Could you check a few things on this drawing? It's one solid part, dimensions in mm from its lowest x, y, z. A direction names the side the tool comes from. Round coordinates to 2 decimals unless told otherwise and drop trailing zeros. Write each loop counter-clockwise with the first axis right and the second up, starting at its lowest first coordinate (ties: lowest second). Pieces come first, ordered by that corner, then holes. Notation, with made-up numbers: (-2.5, 21) -> (11.5, 21) arc R7 cw to (11.5, 26) -> close; hole circle Ø8 at (-22.5, -23.75). An arc over 180 degrees is marked (long way). Put each result on its own line as item: value. Start each with the question number.
1) If I drill on line 1 along Y through (x, z) = (31, 18); line 2 along X through (y, z) = (3.5, 12.5), over which ranges is the centre line in solid material (lowest first)? Write a range as [from, to].
2) I want a section at A-A, the plane y = 8.5. List the corners of the cut face in (x, z) for me, then the cut area to 3 significant figures.
3) I want a section at B-B, the plane z = 12.5. List the corners of the cut face in (x, y) for me.
4) Which directions (+Z, -Z, +X, -X, +Y, -Y) give clear straight access to the entire face, cutting with the end or side of a thin tool? Please do the marked faces 4 and 5.
5) I want a section at D-D, the plane y = 25. List the corners of the cut face in (x, z) for me, then the cut area to 3 significant figures.
6) We'd pull the mould along X, two halves only. Please class the marked faces 1, 2 and 3: released by +X, released by -X, zero draft, split by the parting line, or undercut.
7) Will this pin go through, and if not, where does the flat tip stop? P1, Ø1, axis at x = 36, z = 6, coming from the -Y side.
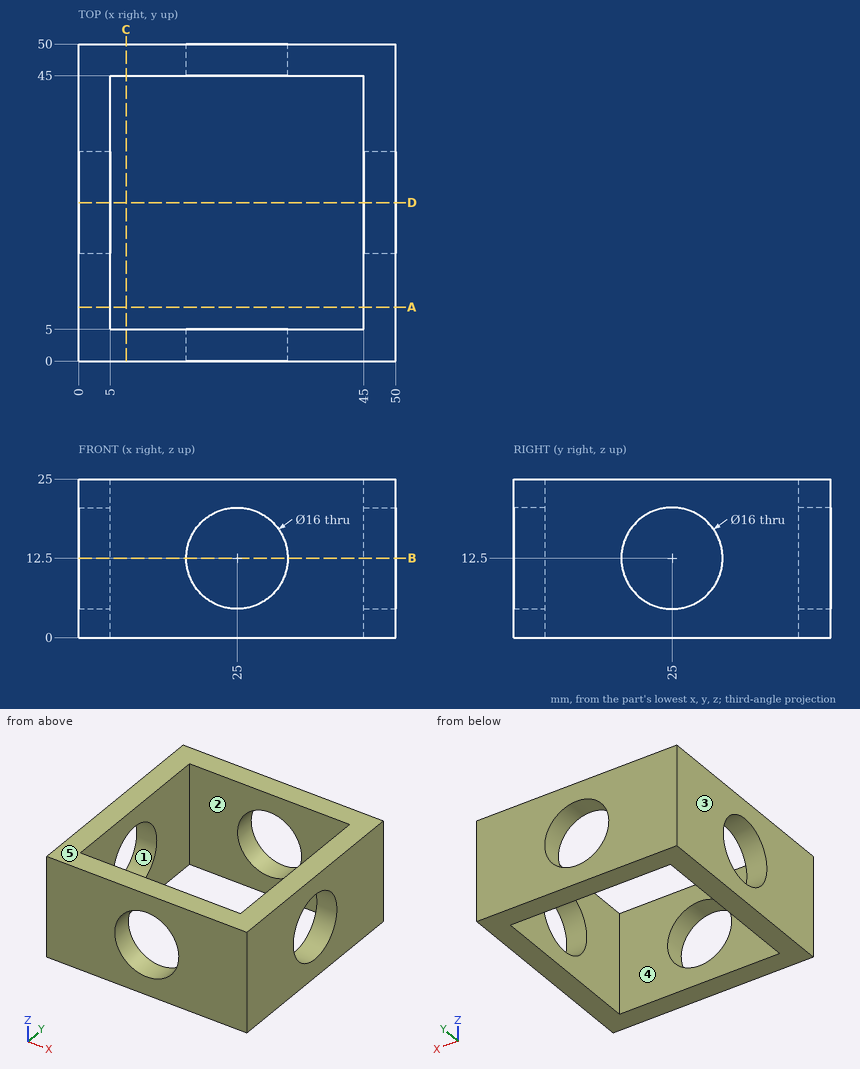
Findings:
1. line 1: y = [0, 5], [45, 50]
1. line 2: x = [0, 17], [33, 50]
2. outline: (0, 0) -> (5, 0) -> (5, 25) -> (0, 25) -> close; (45, 0) -> (50, 0) -> (50, 25) -> (45, 25) -> close
2. area: 250 mm2
3. outline: (0, 0) -> (17, 0) -> (17, 5) -> (5, 5) -> (5, 17) -> (0, 17) -> close; (0, 33) -> (5, 33) -> (5, 45) -> (17, 45) -> (17, 50) -> (0, 50) -> close; (33, 0) -> (50, 0) -> (50, 17) -> (45, 17) -> (45, 5) -> (33, 5) -> close; (33, 45) -> (45, 45) -> (45, 33) -> (50, 33) -> (50, 50) -> (33, 50) -> close
4. face 4: +Z, -Z
4. face 5: +Z, +X, -X, +Y, -Y
5. outline: (0, 0) -> (5, 0) -> (5, 4.5) -> (0, 4.5) -> close; (0, 20.5) -> (5, 20.5) -> (5, 25) -> (0, 25) -> close; (45, 0) -> (50, 0) -> (50, 4.5) -> (45, 4.5) -> close; (45, 20.5) -> (50, 20.5) -> (50, 25) -> (45, 25) -> close
5. area: 90.0 mm2
6. face 1: zero draft
6. face 2: undercut
6. face 3: released by -X
7. P1: stops at y = 0
